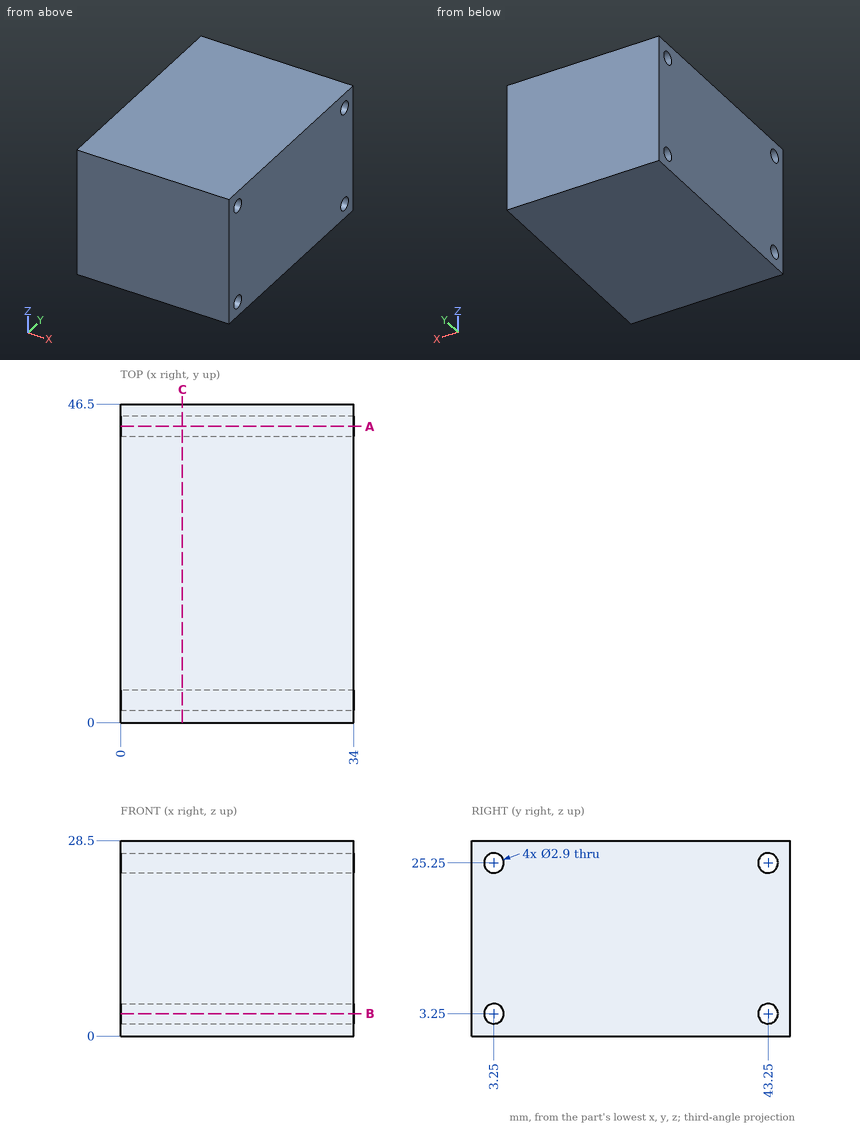
Geometry: see drawing. Coordinates: mm, zero at the bounding-box minimum. Round coordinates to 2 decimals unless told otherwise and drop trailing zeros. Order: outer loops, then holes, each group sorted by start corner. A loop starts at its lowest first (then second) coordinate and runs counter-clockwise, first axis right, second up. Notation, with made-up numbers: (48.25, 84.25) - (105.25, 84.25) arc R22 cw to (105.25, 95.25) - close; hole circle Ø4 at (22, 1.25). An arc over 180 degrees is marked (long way). Use a Markdown table: item, result. Add a question column.
1. Section query A-A (y = 43.25). Return the cut outline in (x, z).
2. Section query B-B (z = 3.25). Return the cut outline in (x, y), then the cut area to 3 significant figures.
3. First-contact query: pin 1 (1.7 mm diameter, centred on y = 43.25, z = 25.25, fed in from -X); pin 2 (4.5 mm diameter, centred on y = 43.25, z = 3.25, fed in from +X). Flat tips, straight axial feed; report the tip coordinate or a pass-through.
4. Section query C-C (x = 9). Return the cut outline in (y, z).
5. Line query: probe 1 along Z at (x, y) = (25.5, 43.25). Output: solid intervals per line, ascending.
Derived:
| question | item | result |
|---|---|---|
| 1 | outline | (0, 0) - (34, 0) - (34, 1.8) - (0, 1.8) - close; (0, 4.7) - (34, 4.7) - (34, 23.8) - (0, 23.8) - close; (0, 26.7) - (34, 26.7) - (34, 28.5) - (0, 28.5) - close |
| 2 | outline | (0, 0) - (34, 0) - (34, 1.8) - (0, 1.8) - close; (0, 4.7) - (34, 4.7) - (34, 41.8) - (0, 41.8) - close; (0, 44.7) - (34, 44.7) - (34, 46.5) - (0, 46.5) - close |
| 2 | area | 1,380 mm2 |
| 3 | pin 1 | through |
| 3 | pin 2 | x = 34 |
| 4 | outline | (0, 0) - (46.5, 0) - (46.5, 28.5) - (0, 28.5) - close; hole circle Ø2.9 at (3.25, 3.25); hole circle Ø2.9 at (3.25, 25.25); hole circle Ø2.9 at (43.25, 3.25); hole circle Ø2.9 at (43.25, 25.25) |
| 5 | probe 1 | 0 to 1.8, 4.7 to 23.8, 26.7 to 28.5 |
